Can you work these out from the model? Positions are in its coordinate system, mm. A direction names the side the tool comes from. Round coordinates to 2 decimals unless told otherwise and drop trailing zeros. Loops run counter-clockwise (first coordinate to the right, second up) from the corner with the lowest first, then second, coordinate; pieces in that order, holes last.
```python
from build123d import *
from build123d import SkipClean  # not in build123d's __all__

# Parameters (mm, degrees)
F2_R      = 3.05
F3_DEPTH  = 13
F4_R      = 0.5
F5_R      = 1.2
F6_DEPTH  = 10
F7_R      = 1.5
F8_DEPTH  = 13
F10_DEPTH = 2.5
F11_DEPTH = 2.5
F13_DEPTH = 2.5


# Not quite as in the source:
# - after a boolean that leaves OpenCascade's solid faulty, fix() repairs it


with BuildPart() as f1:
    # F0 (on Front) → F1 (revolve)
    with BuildSketch(Plane.XZ):
        Polygon((-5, 0), (0, 0), (0, 15), (-8, 15), (-8, 0), align=None)
    revolve(axis=Axis((0, 0, -3.6677676575), (0, 0, -1)))

    # F2 (on face) → F3 (cut)
    with BuildSketch(Plane(origin=(0, 0, 0), x_dir=(1, 0, 0), z_dir=(0, 0, -1))):
        Circle(F2_R)
    extrude(amount=-F3_DEPTH, mode=Mode.SUBTRACT)

    # F4
    f4_edges = [f1.edges().sort_by_distance(p)[0] for p in [
        (8, 0, 15),
    ]]
    fillet(f4_edges, radius=F4_R)

    # F5 (on Front) → F6 (cut)
    with BuildSketch(Plane.XZ):
        with Locations((0, 9)):
            Circle(F5_R)
    extrude(amount=F6_DEPTH, mode=Mode.SUBTRACT)

    # F7 (on face) → F8 (cut)
    with BuildSketch(Plane(origin=(0, 0, 0), x_dir=(1, 0, 0), z_dir=(0, 0, -1))):
        with Locations((-9, 0)):
            Circle(F7_R)
        with Locations((-7.7942286341, -4.5)):
            Circle(F7_R)
        with Locations((-4.5, -7.7942286341)):
            Circle(F7_R)
        with Locations((0, -9)):
            Circle(F7_R)
        with Locations((4.5, -7.7942286341)):
            Circle(F7_R)
        with Locations((7.7942286341, -4.5)):
            Circle(F7_R)
        with Locations((9, 0)):
            Circle(F7_R)
        with Locations((7.7942286341, 4.5)):
            Circle(F7_R)
        with Locations((4.5, 7.7942286341)):
            Circle(F7_R)
        with Locations((0, 9)):
            Circle(F7_R)
        with Locations((-4.5, 7.7942286341)):
            Circle(F7_R)
        with Locations((-7.7942286341, 4.5)):
            Circle(F7_R)
    extrude(amount=-F8_DEPTH, mode=Mode.SUBTRACT)

    # F9 (on face) → F10 (cut)
    with BuildSketch(Plane(origin=(0, 0, 0), x_dir=(1, 0, 0), z_dir=(0, 0, -1))):
        with BuildLine():
            Line((8, 0), (0, 0))
            Line((0, 0), (0, 8))
            ThreePointArc((0, 8), (-5.6568542495, -5.6568542495), (8, 0))
        make_face()
    extrude(amount=-F10_DEPTH, mode=Mode.SUBTRACT)

    # F10_face (on face) + F1_face (on face) → F11 (join)
    with BuildSketch(Plane(origin=(-1.2304392028, 1.2304392022, 2.5), x_dir=(1, 0, 0), z_dir=(0, 0, -1))):
        with BuildLine():
            Line((8.7304392028, 1.2304392022), (4.2804392028, 1.2304392022))
            ThreePointArc((4.2804392028, 1.2304392022), (-0.9262364799, -0.9262364804), (1.2304392028, 4.2804392022))
            Line((1.2304392028, 4.2804392022), (1.2304392028, 8.7304392022))
            ThreePointArc((1.2304392028, 8.7304392022), (0.6621816316, 8.8422449317), (0.1786366634, 9.1609947585))
            ThreePointArc((0.1786366641, 9.1609947578), (-0.8401131581, 8.9578458126), (-1.8239508568, 8.6244030488))
            ThreePointArc((-1.8239508568, 8.6244030488), (-2.5195607972, 7.7256297306), (-3.6457262932, 7.5726005102))
            ThreePointArc((-3.6457262932, 7.5726005102), (-4.4264150467, 6.8872934517), (-5.1117221052, 6.1066046982))
            ThreePointArc((-5.1117221052, 6.1066046982), (-5.2647513256, 4.9804392022), (-6.1635246438, 4.2848292618))
            ThreePointArc((-6.1635246438, 4.2848292618), (-6.4969674076, 3.3009915631), (-6.7001163528, 2.2822417409))
            ThreePointArc((-6.7001163528, 2.2822417409), (-6.2695607972, 1.2304392022), (-6.7001163528, 0.1786366636))
            ThreePointArc((-6.7001163528, 0.1786366636), (-6.4969674076, -0.8401131586), (-6.1635246438, -1.8239508573))
            ThreePointArc((-6.1635246438, -1.8239508573), (-5.2647513256, -2.5195607978), (-5.1117221052, -3.6457262937))
            ThreePointArc((-5.1117221052, -3.6457262937), (-4.4264150467, -4.4264150472), (-3.6457262932, -5.1117221057))
            ThreePointArc((-3.6457262932, -5.1117221057), (-2.5195607972, -5.2647513261), (-1.8239508568, -6.1635246443))
            ThreePointArc((-1.8239508568, -6.1635246443), (-0.8401131581, -6.4969674081), (0.1786366641, -6.7001163533))
            ThreePointArc((0.1786366641, -6.7001163533), (1.2304392028, -6.2695607978), (2.2822417414, -6.7001163533))
            ThreePointArc((2.2822417414, -6.7001163533), (3.3009915636, -6.4969674081), (4.2848292623, -6.1635246443))
            ThreePointArc((4.2848292623, -6.1635246443), (4.9804392028, -5.2647513261), (6.1066046987, -5.1117221057))
            ThreePointArc((6.1066046987, -5.1117221057), (6.8872934522, -4.4264150472), (7.5726005107, -3.6457262937))
            ThreePointArc((7.5726005107, -3.6457262937), (7.7256297311, -2.5195607978), (8.6244030493, -1.8239508573))
            ThreePointArc((8.6244030493, -1.8239508573), (8.9578458131, -0.8401131586), (9.1609947583, 0.1786366636))
            ThreePointArc((9.1609947583, 0.1786366636), (8.842244932, 0.6621816315), (8.7304392028, 1.2304392022))
        make_face()
    with BuildSketch(Plane(origin=(0, 0, 0), x_dir=(1, 0, 0), z_dir=(0, 0, -1))):
        with BuildLine():
            ThreePointArc((1.0518025386, 7.9305555556), (0.5682575707, 7.6118057293), (0, 7.5))
            Line((0, 7.5), (0, 3.05))
            ThreePointArc((0, 3.05), (2.1566756826, 2.1566756826), (3.05, 0))
            Line((3.05, 0), (7.5, 0))
            ThreePointArc((7.5, 0), (7.6118057293, 0.5682575707), (7.9305555556, 1.0518025386))
            ThreePointArc((7.9305555556, 1.0518025386), (7.7274066103, 2.0705523608), (7.3939638465, 3.0543900596))
            ThreePointArc((7.3939638465, 3.0543900596), (6.4951905284, 3.75), (6.3421613079, 4.876165496))
            ThreePointArc((6.3421613079, 4.876165496), (5.6568542495, 5.6568542495), (4.876165496, 6.3421613079))
            ThreePointArc((4.876165496, 6.3421613079), (3.75, 6.4951905284), (3.0543900596, 7.3939638465))
            ThreePointArc((3.0543900596, 7.3939638465), (2.0705523608, 7.7274066103), (1.0518025386, 7.9305555556))
        make_face()
    with SkipClean():  # cleaning this boolean's faces spoils the solid; the shape is the same uncleaned
        extrude(amount=F11_DEPTH)

    # F12 (on face) → F13 (cut)
    with BuildSketch(Plane(origin=(0, 0, -2.5), x_dir=(1, 0, 0), z_dir=(0, 0, -1))):
        with BuildLine():
            ThreePointArc((0, 3.05), (2.1566756826, 2.1566756826), (3.05, 0))
            Line((3.05, 0), (5.35, 0))
            ThreePointArc((5.35, 0), (3.7410791492, 3.7410791492), (0, 5.35))
            Line((0, 5.35), (0, 3.05))
        make_face()
    extrude(amount=-F13_DEPTH, mode=Mode.SUBTRACT)

    add(f1.part.fix(), mode=Mode.REPLACE)


solid = f1.part
```
(1) Which directions (+Z, -Z, +X, -X, +Y, -Y) give clear straight access to the entire face, cutting with the end or side of a thin tool? Please do faces 4 (the flat face through (-4, 0, 0)), 5 (the cylindrical face through (0, -7.5, 11.6)), 6 (the cylindrical face through (-0.16, -5.33, 10.19)).
(2) Suppose I cut it at B-B (z = -0.5). Write out the boundary of the cut face in (x, y).
(3) We'd pull the mould along X, two halves only. Please class faces 1 (the flat face through (0, 0, 13)), 2 (the flat face through (-6.8, -3.9, 13)), 3 (the flat face through (0, -6, -1)): released by +X, released by -X, zero draft, split by the parting line, or undercut.
(4) For pin 1 (0.9 mm diameter, centred on x = -7, y = 4, fed in from -Z); pin 2 (6 mm diameter, centred on x = -6, z = 13, fed in from +Y); pin 3 (4 mm diameter, centred on y = 3.5, z = 2, fed in from +X), each with a flat end and sliding along its axis, tell me the tip position at first contact or that it passes through.
(5) Suppose I cut it at C-C (z = 9). Write out the boundary of the cut face in (x, y), then the cut area to 3 significant figures.
(6) If I drill on line 1 (X direction, y = 0, z = 6.75); line 2 (Z direction, x = -3, y = -1), over which ranges is the centre line in solid material (lowest first)?
(7) Suppose I cut it at A-A (z = 12.75). Write out the boundary of the cut face in (x, y), then the cut area to 3 significant figures.
Check result:
1. face 4: -Z, -X, +Y
1. face 5: -Z, -Y
1. face 6: -Y
2. outline: (0, -7.5) arc R1.5 cw to (1.05, -7.93) arc R8 ccw to (3.05, -7.39) arc R1.5 cw to (4.88, -6.34) arc R8 ccw to (6.34, -4.88) arc R1.5 cw to (7.39, -3.05) arc R8 ccw to (7.93, -1.05) arc R1.5 cw to (7.5, 0) - (5.35, 0) arc R5.5 cw to (0, -5.35) - close
3. face 1: undercut
3. face 2: zero draft
3. face 3: released by -X
4. pin 1: stops at z = 13
4. pin 2: stops at y = 7.42
4. pin 3: stops at x = 7.86
5. outline: (-7.93, -1.05) arc R8 ccw to (-7.39, -3.05) arc R1.5 cw to (-6.34, -4.88) arc R8 ccw to (-4.88, -6.34) arc R1.5 cw to (-3.05, -7.39) arc R8 ccw to (-1.2, -7.91) - (-1.2, -2.8) arc R3.05 cw (long way) to (1.2, -2.8) - (1.2, -7.91) arc R8 ccw to (3.05, -7.39) arc R1.5 cw to (4.88, -6.34) arc R8 ccw to (6.34, -4.88) arc R1.5 cw to (7.39, -3.05) arc R8 ccw to (7.93, -1.05) arc R1.5 cw to (7.93, 1.05) arc R8 ccw to (7.39, 3.05) arc R1.5 cw to (6.34, 4.88) arc R8 ccw to (4.88, 6.34) arc R1.5 cw to (3.05, 7.39) arc R8 ccw to (1.05, 7.93) arc R1.5 cw to (-1.05, 7.93) arc R8 ccw to (-3.05, 7.39) arc R1.5 cw to (-4.88, 6.34) arc R8 ccw to (-6.34, 4.88) arc R1.5 cw to (-7.39, 3.05) arc R8 ccw to (-7.93, 1.05) arc R1.5 cw to start
5. area: 152 mm2
6. line 1: x = -7.5 to -3.05, 3.05 to 7.5
6. line 2: z = 0 to 15
7. outline: (-7.93, -1.05) arc R8 ccw to (-7.39, -3.05) arc R1.5 cw to (-6.34, -4.88) arc R8 ccw to (-4.88, -6.34) arc R1.5 cw to (-3.05, -7.39) arc R8 ccw to (-1.05, -7.93) arc R1.5 cw to (1.05, -7.93) arc R8 ccw to (3.05, -7.39) arc R1.5 cw to (4.88, -6.34) arc R8 ccw to (6.34, -4.88) arc R1.5 cw to (7.39, -3.05) arc R8 ccw to (7.93, -1.05) arc R1.5 cw to (7.93, 1.05) arc R8 ccw to (7.39, 3.05) arc R1.5 cw to (6.34, 4.88) arc R8 ccw to (4.88, 6.34) arc R1.5 cw to (3.05, 7.39) arc R8 ccw to (1.05, 7.93) arc R1.5 cw to (-1.05, 7.93) arc R8 ccw to (-3.05, 7.39) arc R1.5 cw to (-4.88, 6.34) arc R8 ccw to (-6.34, 4.88) arc R1.5 cw to (-7.39, 3.05) arc R8 ccw to (-7.93, 1.05) arc R1.5 cw to start; hole circle Ø6.1 at (0, 0)
7. area: 163 mm2
